from build123d import *

# Parameters (mm, degrees)
SKETCH028_W              = 37
SKETCH028_H              = 8
SKETCH028_R              = 1.75
PAD016_DEPTH             = 3
PAD017_DEPTH             = 8.4
SKETCH030_R              = 10
PAD018_DEPTH             = 20
SKETCH031_R              = 1.920563
PAD019_DEPTH             = 2
SKETCH032_R              = 1.5
PAD020_DEPTH             = 10
BODY008_ROLL_ANGLE       = -90
BODY008_PITCH_ANGLE      = -30
BODY008_PLACEMENT_ANGLE  = 180
CLONE001_PLACEMENT_ANGLE = 210
BODY009_PLACEMENT_ANGLE  = 45


with BuildPart() as part:
    # Sketch028 → Pad016 (new body)
    with BuildSketch(Plane.XY):
        Rectangle(SKETCH028_W, SKETCH028_H)
        with Locations((15.456405, 0)):
            Circle(SKETCH028_R, mode=Mode.SUBTRACT)
        with Locations((-15.543595, 0)):
            Circle(SKETCH028_R, mode=Mode.SUBTRACT)
    extrude(amount=-PAD016_DEPTH)

    # Sketch029 → Pad017 (join)
    with BuildSketch(Plane.XY):
        with BuildLine():
            ThreePointArc((-11.652801, 4.52352), (-7.163489, -10.243751), (8.24762, -9.392911))
            ThreePointArc((8.24762, -9.392911), (12.786665, -8.95332), (11.647301, -4.537663))
            ThreePointArc((11.647301, -4.537663), (7.175919, 10.235047), (-8.236211, 9.402916))
            ThreePointArc((-8.236211, 9.402916), (-12.696857, 8.890435), (-11.652801, 4.52352))
        make_face()
    extrude(amount=-PAD017_DEPTH)

    # Sketch030 → Pad018 (join)
    with BuildSketch(Plane.XY):
        Circle(SKETCH030_R)
    extrude(amount=-PAD018_DEPTH)

    # Sketch031 → Pad019 (join)
    with BuildSketch(Plane.XY):
        with Locations((0, 6)):
            Circle(SKETCH031_R)
    extrude(amount=PAD019_DEPTH)

    # Sketch032 → Pad020 (join)
    with BuildSketch(Plane.XY):
        with Locations((0, 6.01563)):
            Circle(SKETCH032_R)
    extrude(amount=PAD020_DEPTH)


with BuildPart() as part_1:
    # Body008 roll: moved
    add(part.part.rotate(Axis((0, 0, 0), (1, 0, 0)), BODY008_ROLL_ANGLE))


with BuildPart() as part_2:
    # Body008 pitch: moved
    add(part_1.part.rotate(Axis((0, 0, 0), (0, 1, 0)), BODY008_PITCH_ANGLE))


with BuildPart() as part_3:
    # Body008 placement: moved
    add(part_2.part.moved(Location((-56.598076, 17, -9.800515))).rotate(Axis((-56.598076, 17, -9.800515), (0, 0, 1)), BODY008_PLACEMENT_ANGLE))


with BuildPart() as part_4:
    # Clone001 placement: moved
    add(part_3.part.moved(Location((-103.715114, 0, -57.786533))).rotate(Axis((-103.715114, 0, -57.786533), (0, -1, 0)), CLONE001_PLACEMENT_ANGLE))


with BuildPart() as part_5:
    # Body009 placement: moved
    add(part_4.part.moved(Location((0.05412, 8, 13.784986))).rotate(Axis((0.05412, 8, 13.784986), (0, 1, 0)), BODY009_PLACEMENT_ANGLE))


solid = part_5.part
Geometry check sheet. Reference: the model listing, model coordinates, mm. A direction names the side the tool comes from. Give positions to 0.01 mm unless a question says otherwise; leave off trailing zeros. Order: outer loops, then holes, each group sorted by start corner. A loop starts at its lowest first (then second) coordinate and runs counter-clockwise, first axis right, second up.
1. Sectioned sample at A-A (z = 54.5). Record the boundary of the cut face in (x, y), then the cut area to 3 significant figures.
Completed:
outline: (-69.68, 25) - (-64.7, 25) - (-64.7, 28) - (-69.68, 28) - close; (-61.9, 25) - (-56.32, 25) - (-56.32, 33.4) - (-61.9, 33.4) - close
area: 61.8 mm2
2. Sectioned sample at C-C (x = -65.5). Record the boundary of the cut face in (y, z), then the cut area to 3 significant figures.
Completed:
outline: (25, 31.97) - (33.4, 31.97) - (33.4, 35.91) - (45, 35.91) - (45, 46.25) - (33.4, 46.25) - (33.4, 50.19) - (28, 50.19) - (28, 55.3) - (25, 55.3) - close
area: 288 mm2
3. Draft check along X on faces 1 (the face through (-54.316, 24.014, 44.291)), 2 (the face through (-54.3, 29.141, 25.695)), 3 (the face through (-45, 28, 32)). Enter one of: pulls with the +X half, pulls with the -X half, needs draft (parallel to the pull), parting line crosses it, or undercut.
Completed:
face 1: parting line crosses it
face 2: undercut
face 3: needs draft
4. Sectioned sample at D-D (z = 48). Record the boundary of the cut face in (x, y).
Completed:
outline: (-69.52, 25) - (-46.53, 25) - (-46.53, 33.4) - (-49.72, 33.4) - (-49.72, 45) - (-64.16, 45) - (-64.16, 33.4) - (-67.35, 33.4) - (-67.35, 28) - (-69.52, 28) - close
5. Scan lines: line 1 (Y direction, x = -47.5, z = 33); line 2 (Y direction, x = -55, z = 36); line 3 (Z direction, x = -66.5, y = 26). Record each from-to range of solid material in increasing order.
Completed:
line 1: y = 25 to 33.4
line 2: y = 25 to 45
line 3: z = 33.03 to 51.06, 53.08 to 56.3
6. Sectioned sample at B-B (y = 26.5). Record the boundary of the cut face in (x, z), then the cut area to 3 significant figures.
Completed:
outline: (-72.85, 51.33) - (-68.14, 46.62) arc R12.5 ccw to (-57.75, 28.61) arc R3 ccw (long way) to (-51.91, 29.63) arc R12.5 ccw to (-51.39, 29.88) - (-46.69, 25.17) - (-41.03, 30.83) - (-45.74, 35.53) arc R12.5 ccw to (-56.11, 53.55) arc R3 ccw (long way) to (-61.98, 52.52) arc R12.5 ccw to (-62.48, 52.28) - (-67.19, 56.99) - close; hole circle Ø3.5 at (-67.93, 52.07); hole circle Ø3.5 at (-46.01, 30.15)
area: 601 mm2
7. Depth check by flat-ended pin: pin 1 (3 mm diameter, centred on x = -47, z = 29.5, fed in from +Y); pin 2 (8 mm diameter, centred on x = -66.5, z = 53.5, fed in from -Y); pin 3 (8 mm diameter, centred on x = -66.5, y = 29, fed in from -Z); pin 4 (5 mm diameter, centred on x = -65, z = 49.5, fed in from +Y). Enter the tip coordinate at first touch or a pass-through.
Completed:
pin 1: stops at y = 28
pin 2: stops at y = 25
pin 3: stops at z = 29.88
pin 4: stops at y = 45
8. Access from +Z, -Z, +X, -X, +Y, -Y to the whole of each face (thin tool, end or side, straight path). Record for faces 4 (the face through (-64.9, 26.5, 54.7)), 5 (the face through (-53.7, 19.06, 46.44)), 6 (the face through (-59.949, 39.119, 31.543)), 7 (the face through (-70.528, 26.479, 49.012)), 8 (the face through (-49.072, 26.479, 27.556)).
Completed:
face 4: +Z, +Y, -Y
face 5: -Y
face 6: +Y
face 7: -X, +Y, -Y
face 8: -Z, +Y, -Y
